Geometry check sheet. Reference: the model listing, model coordinates, mm. A direction names the side the tool comes from. Round coordinates to 2 decimals unless told otherwise and drop trailing zeros. Loops run counter-clockwise (first coordinate to the right, second up) from the corner with the lowest first, then second, coordinate; pieces in that order, holes last. Notation, with made-up numbers: (-21.5, 62) -> (-17.5, 62) arc R20 ccw to (-17.5, 67) -> close; hole circle Ø1 at (-21, -32.5). An arc over 180 degrees is marked (long way). Use one line per item in the form item = value.
Autodesk Inventor part; units mm, degrees
ref_plane "YZ Plane" through (0, 0, 0) normal (1, 0, 0) x (0, 1, 0)
ref_plane "XZ Plane" through (0, 0, 0) normal (0, 1, 0) x (-1, 0, 0)
ref_plane "XY Plane" through (0, 0, 0) normal (0, 0, 1) x (1, 0, 0)
sketch "草圖1" plane through (0, 0, 0) normal (0, 1, 0) x (-1, 0, 0)
  line L0 (-33.5, 27) -> (33.5, 27)
  line L1 (33.5, 27) -> (33.5, -27)
  line L2 (33.5, -27) -> (-33.5, -27)
  line L3 (-33.5, -27) -> (-33.5, 27)
  line L4 (-33.5, 27) -> (33.5, -27) construction
  line L5 (33.5, 27) -> (-33.5, -27) construction
  line L6 (43.5, -4.5) -> (33.5, -4.5)
  line L7 (33.5, -4.5) -> (33.5, 4.5)
  line L8 (33.5, 4.5) -> (43.5, 4.5)
  line L9 (43.5, 4.5) -> (43.5, -4.5)
  line L10 (-33.5, -4.5) -> (-43.5, -4.5)
  line L11 (-43.5, -4.5) -> (-43.5, 4.5)
  line L12 (-43.5, 4.5) -> (-33.5, 4.5)
  line L13 (-33.5, 4.5) -> (-33.5, -4.5)
  point P0 (0, 0)
  point P1 (33.5, 0)
  point P2 (-33.5, 0)
  point P3 (-33.5, 4.5)
  point P4 (-33.5, -4.5)
  dimension "d0" = 67
  dimension "d1" = 54
  dimension "d2" = 9
  dimension "d3" = 10
extrude "擠出1" add sketch "草圖1" along normal blind 150
sketch "草圖2" plane through (-33.5, 0, 27) normal (0, 0, 1) x (1, 0, 0)
  line L0 (0, 0) -> (0, 150)
  line L1 (0, 150) -> (67, 150)
  line L2 (67, 150) -> (67, 0)
  line L3 (67, 0) -> (0, 0)
  circle A0 centre (33.5, 56) radius 30
  line L4 (3.5, 56) -> (63.5, 56)
  line L5 (63.5, 56) -> (63.5, -16.9471)
  line L6 (63.5, -16.9471) -> (3.5, -16.9471)
  line L7 (3.5, -16.9471) -> (3.5, 56)
  point P0 (33.5, 0)
  point P1 (33.5, 0)
  point P2 (3.5, 56)
  dimension "d6" = 60
  dimension "d7" = 56
extrude "擠出2" cut sketch "草圖2" against normal through all contours L7 A0 L5 L3 | L3 L5 L6 L7 | L4 A0 | A0 L4
sketch "草圖3" plane through (33.5, 150, -27) normal (0, 0, -1) x (-1, 0, 0)
  arc A0 (63.5, -94) -> (3.5, -94) centre (33.5, -94) ccw construction
  circle A1 centre (33.5, -90) radius 30
  line L0 (63.5, -150) -> (3.5, -150)
  line L1 (3.5, -150) -> (3.5, -90)
  line L2 (3.5, -90) -> (63.5, -90)
  line L3 (63.5, -90) -> (63.5, -150)
  point P0 (33.5, -150)
  point P1 (33.5, -150)
  point P2 (63.5, -150)
  dimension "d10" = 60
  dimension "d11" = 4
sketch "草圖4" plane through (-33.5, 150, 27) normal (0, 0, 1) x (1, 0, 0)
  arc A0 (63.5, -94) -> (3.5, -94) centre (33.5, -94) ccw construction
  circle A1 centre (33.5, -88) radius 30
  line L0 (63.5, -150) -> (3.5, -150)
  line L1 (3.5, -150) -> (3.5, -88)
  line L2 (3.5, -88) -> (63.5, -88)
  line L3 (63.5, -88) -> (63.5, -150)
  point P0 (33.5, -150)
  dimension "d12" = 6
  dimension "d13" = 60
loft "斷面混成1" cut profiles "草圖3", "草圖4"
properties part number "Slider-2"
1. Section check C-C (x = -38). Record the boundary of the cut face in (y, z), then the cut area to 3 significant figures.
Return value:
outline = (0, -4.5) -> (150, -4.5) -> (150, 4.5) -> (0, 4.5) -> close
area = 1,350 mm2
2. Section check A-A (y = 33). Record the boundary of the cut face in (x, z).
Return value:
outline = (-43.5, -4.5) -> (-33.5, -4.5) -> (-33.5, -27) -> (-30, -27) -> (-30, 27) -> (-33.5, 27) -> (-33.5, 4.5) -> (-43.5, 4.5) -> close; (30, -27) -> (33.5, -27) -> (33.5, -4.5) -> (43.5, -4.5) -> (43.5, 4.5) -> (33.5, 4.5) -> (33.5, 27) -> (30, 27) -> close
3. Material ranges on line 1 along X through (y, z) = (19.5, -19); line 2 along X through (y, z) = (93, -8.5); line 3 along Z through (x, y) = (-39, 85), recorded low to high.
Return value:
line_1 = -33.5 to -30, 30 to 33.5
line_2 = -33.5 to 33.5
line_3 = -4.5 to 4.5
4. Gauge pin test, flat ends, axial feed: pin 1 (7 mm diameter, centred on y = 65, z = -15, fed in from -X); pin 2 (25 mm diameter, centred on y = 47, z = -18, fed in from +X); pin 3 (5 mm diameter, centred on x = 37, y = 93.5, fed in from +Z). Record the tip position at first contact, or that the pin passes through.
Return value:
pin_1 = -33.5
pin_2 = 33.5
pin_3 = 4.5
5. Tool access check on faces 4 (the flat face through (38, 74, -4.5)), 5 (the flat face through (39, 74, 4.5)), 6 (the flat face through (-39, 74, -4.5)). Record the directions out of +Z, -Z, +X, -X, +Y, -Y that give a thin tool (end or side, any length) a straight path to the whole face; none if there is none.
Return value:
face_4 = -Z, +X, +Y, -Y
face_5 = +Z, +X, +Y, -Y
face_6 = -Z, -X, +Y, -Y
6. Mould release check, pull along X, two halves, no side actions. Record for faces 1 (the flat face through (-33.5, 74, -16)), 2 (the flat face through (43.5, 74, 0)), 3 (the flat face through (-30, 31, 0)): released by +X, released by -X, zero draft, split by the parting line, or undercut.
Return value:
face_1 = released by -X
face_2 = released by +X
face_3 = undercut
7. Section check B-B (y = 117.5). Record the boundary of the cut face in (x, z).
Return value:
outline = (-43.5, -4.5) -> (-33.5, -4.5) -> (-33.5, -27) -> (33.5, -27) -> (33.5, -4.5) -> (43.5, -4.5) -> (43.5, 4.5) -> (33.5, 4.5) -> (33.5, 27) -> (-33.5, 27) -> (-33.5, 4.5) -> (-43.5, 4.5) -> close
